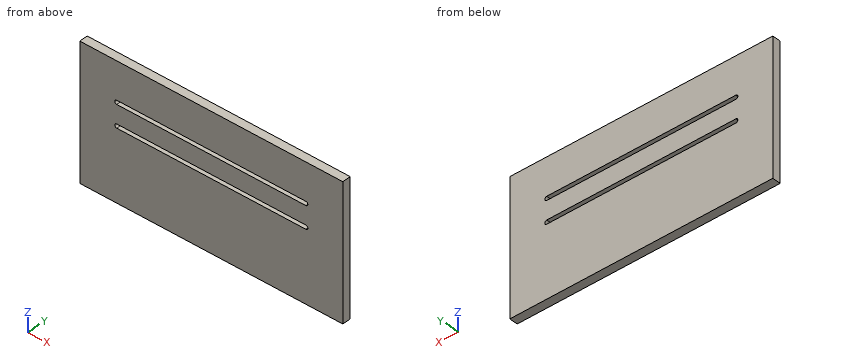
```python
from build123d import *

# Parameters (mm, degrees)
SKETCH1_W           = 298.45
SKETCH1_H           = 152.4
BOSS_EXTRUDE1_DEPTH = 4.7625
CUT_EXTRUDE2_DEPTH  = 168.825106137


with BuildPart() as part:
    # Sketch1 → Boss-Extrude1 (new, symmetric)
    with BuildSketch(Plane(origin=(0, 0, 0), x_dir=(1, 0, 0), z_dir=(0, 1, 0))):
        Rectangle(SKETCH1_W, SKETCH1_H)
    extrude(amount=BOSS_EXTRUDE1_DEPTH, both=True)

    # Sketch4 → Cut-Extrude2 (cut, through all)
    with BuildSketch(Plane.XZ.offset(4.7625)):
        with BuildLine():
            Line((-107.315, 33.9979), (107.315, 33.9979))
            ThreePointArc((107.315, 33.9979), (109.5629, 31.75), (107.315, 29.5021))
            Line((107.315, 29.5021), (-107.315, 29.5021))
            ThreePointArc((-107.315, 29.5021), (-109.5629, 31.75), (-107.315, 33.9979))
        make_face()
        with BuildLine():
            Line((-107.315, 8.5979), (107.315, 8.5979))
            ThreePointArc((107.315, 8.5979), (109.5629, 6.35), (107.315, 4.1021))
            Line((107.315, 4.1021), (-107.315, 4.1021))
            ThreePointArc((-107.315, 4.1021), (-109.5629, 6.35), (-107.315, 8.5979))
        make_face()
    extrude(amount=-CUT_EXTRUDE2_DEPTH, mode=Mode.SUBTRACT)


solid = part.part
```
Input: part model. Units: mm. Frame: model coordinates. Give positions to 0.01 mm unless a question says otherwise; leave off trailing zeros. Order: outer loops, then holes, each group sorted by start corner. A loop starts at its lowest first (then second) coordinate and runs counter-clockwise, first axis right, second up.
1. Section A-A on x = 37. Return the cut outline in (y, z), and give its area (3 significant figures).
Derived:
outline: (-4.76, -76.2) - (4.76, -76.2) - (4.76, 4.1) - (-4.76, 4.1) - close; (-4.76, 8.6) - (4.76, 8.6) - (4.76, 29.5) - (-4.76, 29.5) - close; (-4.76, 34) - (4.76, 34) - (4.76, 76.2) - (-4.76, 76.2) - close
area: 1,370 mm2
2. Section B-B on y = 1.25. Return the cut outline in (x, z) (3 decimals), and give its area (3 significant figures).
Derived:
outline: (-149.225, -76.2) - (149.225, -76.2) - (149.225, 76.2) - (-149.225, 76.2) - close; hole (-107.315, 4.102) - (107.315, 4.102) arc R2.248 ccw to (107.315, 8.598) - (-107.315, 8.598) arc R2.248 ccw to start; hole (-107.315, 29.502) - (107.315, 29.502) arc R2.248 ccw to (107.315, 33.998) - (-107.315, 33.998) arc R2.248 ccw to start
area: 43,500 mm2
3. Material intervals for L1, parallel to Z at x = -77, y = 3.5, sorted ascending.
Derived:
L1: z = -76.2 to 4.1, 8.6 to 29.5, 34 to 76.2
